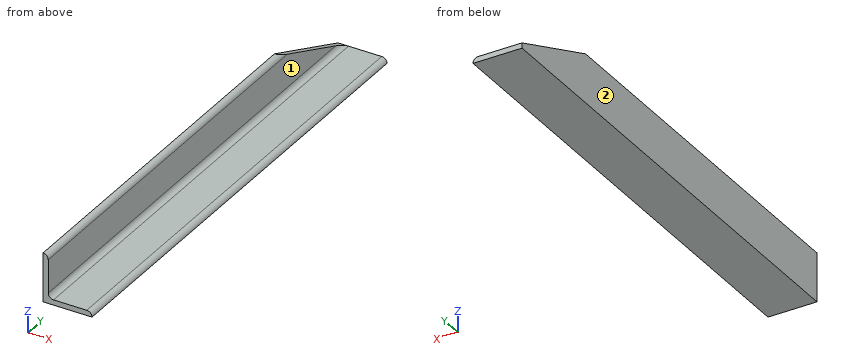
from build123d import *

# Parameters (mm, degrees)
F0_W     = 4.7625
F0_H     = 4.7625
F0_H_2   = 39.6875
F0_W_2   = 39.6875
F1_DEPTH = 222.25
F2_R     = 4.76249
F4_DEPTH = 25.4


# Not quite as in the source:
# - a fillet or chamfer is up to 0.001 mm smaller than in the source, because OpenCascade refuses the exact size


with BuildPart() as f1:
    # F0 (on Front) → F1 (new body, symmetric)
    with BuildSketch(Plane.XZ):
        with Locations((2.38125, 2.38125)):
            Rectangle(F0_W, F0_H)
        with Locations((2.38125, 24.60625)):
            Rectangle(F0_W, F0_H_2)
        with Locations((24.60625, 2.38125)):
            Rectangle(F0_W_2, F0_H)
    extrude(amount=F1_DEPTH, both=True)

    # F2 (radius 4.7625 in the source; OpenCascade refuses exactly that, so slightly less here)
    f2_edges = [f1.edges().sort_by_distance(p)[0] for p in [
        (4.7625, 0, 4.7625),
        (4.7625, 0, 44.45),
        (44.45, 0, 4.7625),
    ]]
    fillet(f2_edges, radius=F2_R)

    # F3 (on face) → F4 (cut)
    with BuildSketch(Plane(origin=(0, 0, 0), x_dir=(0, -1, 0), z_dir=(-1, 0, 0))):
        Polygon((-222.25, 44.45), (-222.25, 4.7625), (-126.4358992433, 44.45), align=None)
    extrude(amount=-F4_DEPTH, mode=Mode.SUBTRACT)


solid = f1.part
CAD build for the part. Positions are in the model's coordinates, mm. Face numbers are marked on the shaded views. A direction names the side the tool comes from. Coordinates: 2 decimals unless noted, no trailing zeros. Loops run counter-clockwise (first coordinate to the right, second up) from the corner with the lowest first, then second, coordinate; pieces in that order, holes last. Notation, with made-up numbers: (51.25, 58.5) -> (93.25, 58.5) arc R30 ccw to (93.25, 95.5) -> close; hole circle Ø11 at (-8.5, -24.75). An arc over 180 degrees is marked (long way). One line per item, written item: value.
1. Flat gauge pins, fed straight in: P1, Ø1, axis at x = 9, y = 84.5, coming from the +Z side; P2, Ø15, axis at y = -15, z = 21, coming from the +X side; P3, Ø15, axis at x = 29, y = -22, coming from the +Z side. Where does each tip first touch, or does it go through?
Answers:
P1: stops at z = 4.87
P2: stops at x = 4.76
P3: stops at z = 4.76
2. Drill centre lines: line 1 (Z direction, x = 39.5, y = 116); line 2 (X direction, y = -172.5, z = 6.5). Where is each one in solid material? Low to high. Write a range as [from, to].
Answers:
line 1: z = [0, 4.76]
line 2: x = [0, 5.85]
3. Which spindle directions (+Z, -Z, +X, -X, +Y, -Y) get a long thin tool onto all of the face, cutting with end or side? Do the marked faces 1 and 2. Say none if no direction does.
Answers:
face 1: +Z, +X, +Y, -Y
face 2: +Z, -Z, -X, +Y, -Y
4. Slice it at B-B on x = 30. Write the cut outline in (y, z), and give its area (3 significant figures).
Answers:
outline: (-222.25, 0) -> (222.25, 0) -> (222.25, 4.76) -> (-222.25, 4.76) -> close
area: 2,120 mm^2
